from build123d import *

# Parameters (mm, degrees)
CYLINDER009_R     = 1.75
CYLINDER009_DEPTH = 10
CYLINDER010_R     = 2.5
CYLINDER010_DEPTH = 4
CYLINDER008_R     = 1.75
CYLINDER008_DEPTH = 10
CYLINDER011_R     = 2.5
CYLINDER011_DEPTH = 4
CYLINDER007_R     = 1.75
CYLINDER007_DEPTH = 10
CYLINDER013_R     = 2.5
CYLINDER013_DEPTH = 4
CYLINDER006_R     = 1.75
CYLINDER006_DEPTH = 10
CYLINDER012_R     = 2.5
CYLINDER012_DEPTH = 4
CYLINDER005_R     = 1.75
CYLINDER005_DEPTH = 10
CYLINDER014_R     = 2.5
CYLINDER014_DEPTH = 4
CYLINDER004_R     = 1.75
CYLINDER004_DEPTH = 10
CYLINDER015_R     = 2.5
CYLINDER015_DEPTH = 4
CYLINDER003_R     = 1
CYLINDER003_DEPTH = 10
CYLINDER002_R     = 1
CYLINDER002_DEPTH = 10
CYLINDER001_R     = 1
CYLINDER001_DEPTH = 10
CYLINDER_R        = 1
CYLINDER_DEPTH    = 10
BOX001_W          = 72
BOX001_H          = 25
BOX001_DEPTH      = 10
BOX_W             = 86
BOX_H             = 70
BOX_DEPTH         = 2
CHAMFER_SIZE      = 0.5
CHAMFER001_SIZE   = 0.5


with BuildPart() as cilindro009:
    # Cylinder009 → Cylinder009 (new body)
    with BuildSketch(Plane(origin=(42, 12.5, -3), x_dir=(1, 0, 0), z_dir=(0, 0, 1))):
        Circle(CYLINDER009_R)
    extrude(amount=CYLINDER009_DEPTH)


with BuildPart() as cut011:
    # Cylinder010 → Cylinder010 (new body)
    with BuildSketch(Plane(origin=(42, 12.5, -2), x_dir=(1, 0, 0), z_dir=(0, 0, 1))):
        Circle(CYLINDER010_R)
    extrude(amount=CYLINDER010_DEPTH)

    # Cut011: cut Cilindro009
    add(cilindro009.part, mode=Mode.SUBTRACT)


with BuildPart() as cilindro008:
    # Cylinder008 → Cylinder008 (new body)
    with BuildSketch(Plane(origin=(34.5, 12.5, -3), x_dir=(1, 0, 0), z_dir=(0, 0, 1))):
        Circle(CYLINDER008_R)
    extrude(amount=CYLINDER008_DEPTH)


with BuildPart() as cut012:
    # Cylinder011 → Cylinder011 (new body)
    with BuildSketch(Plane(origin=(34.5, 12.5, -2), x_dir=(1, 0, 0), z_dir=(0, 0, 1))):
        Circle(CYLINDER011_R)
    extrude(amount=CYLINDER011_DEPTH)

    # Cut012: cut Cilindro008
    add(cilindro008.part, mode=Mode.SUBTRACT)


with BuildPart() as cilindro007:
    # Cylinder007 → Cylinder007 (new body)
    with BuildSketch(Plane(origin=(25, 9.5, -3), x_dir=(1, 0, 0), z_dir=(0, 0, 1))):
        Circle(CYLINDER007_R)
    extrude(amount=CYLINDER007_DEPTH)


with BuildPart() as cut013:
    # Cylinder013 → Cylinder013 (new body)
    with BuildSketch(Plane(origin=(25, 9.5, -2), x_dir=(1, 0, 0), z_dir=(0, 0, 1))):
        Circle(CYLINDER013_R)
    extrude(amount=CYLINDER013_DEPTH)

    # Cut013: cut Cilindro007
    add(cilindro007.part, mode=Mode.SUBTRACT)


with BuildPart() as cilindro006:
    # Cylinder006 → Cylinder006 (new body)
    with BuildSketch(Plane(origin=(25, 16.5, -3), x_dir=(1, 0, 0), z_dir=(0, 0, 1))):
        Circle(CYLINDER006_R)
    extrude(amount=CYLINDER006_DEPTH)


with BuildPart() as cut014:
    # Cylinder012 → Cylinder012 (new body)
    with BuildSketch(Plane(origin=(25, 16.5, -2), x_dir=(1, 0, 0), z_dir=(0, 0, 1))):
        Circle(CYLINDER012_R)
    extrude(amount=CYLINDER012_DEPTH)

    # Cut014: cut Cilindro006
    add(cilindro006.part, mode=Mode.SUBTRACT)


with BuildPart() as cilindro005:
    # Cylinder005 → Cylinder005 (new body)
    with BuildSketch(Plane(origin=(15, 12.5, -3), x_dir=(1, 0, 0), z_dir=(0, 0, 1))):
        Circle(CYLINDER005_R)
    extrude(amount=CYLINDER005_DEPTH)


with BuildPart() as cut015:
    # Cylinder014 → Cylinder014 (new body)
    with BuildSketch(Plane(origin=(15, 12.5, -2), x_dir=(1, 0, 0), z_dir=(0, 0, 1))):
        Circle(CYLINDER014_R)
    extrude(amount=CYLINDER014_DEPTH)

    # Cut015: cut Cilindro005
    add(cilindro005.part, mode=Mode.SUBTRACT)


with BuildPart() as cilindro004:
    # Cylinder004 → Cylinder004 (new body)
    with BuildSketch(Plane(origin=(7.5, 12.5, -3), x_dir=(1, 0, 0), z_dir=(0, 0, 1))):
        Circle(CYLINDER004_R)
    extrude(amount=CYLINDER004_DEPTH)


with BuildPart() as cut016:
    # Cylinder015 → Cylinder015 (new body)
    with BuildSketch(Plane(origin=(7.5, 12.5, -2), x_dir=(1, 0, 0), z_dir=(0, 0, 1))):
        Circle(CYLINDER015_R)
    extrude(amount=CYLINDER015_DEPTH)

    # Cut016: cut Cilindro004
    add(cilindro004.part, mode=Mode.SUBTRACT)


with BuildPart() as cilindro003:
    # Cylinder003 → Cylinder003 (new body)
    with BuildSketch(Plane(origin=(83, 67, -1), x_dir=(1, 0, 0), z_dir=(0, 0, 1))):
        Circle(CYLINDER003_R)
    extrude(amount=CYLINDER003_DEPTH)


with BuildPart() as cilindro002:
    # Cylinder002 → Cylinder002 (new body)
    with BuildSketch(Plane(origin=(83, 3, -1), x_dir=(1, 0, 0), z_dir=(0, 0, 1))):
        Circle(CYLINDER002_R)
    extrude(amount=CYLINDER002_DEPTH)


with BuildPart() as cilindro001:
    # Cylinder001 → Cylinder001 (new body)
    with BuildSketch(Plane(origin=(3, 67, -1), x_dir=(1, 0, 0), z_dir=(0, 0, 1))):
        Circle(CYLINDER001_R)
    extrude(amount=CYLINDER001_DEPTH)


with BuildPart() as cilindro:
    # Cylinder → Cylinder (new body)
    with BuildSketch(Plane(origin=(3, 3, -1), x_dir=(1, 0, 0), z_dir=(0, 0, 1))):
        Circle(CYLINDER_R)
    extrude(amount=CYLINDER_DEPTH)


with BuildPart() as cubo001:
    # Box001 → Box001 (new body)
    with BuildSketch(Plane(origin=(7, 25.5, 0), x_dir=(1, 0, 0), z_dir=(0, 0, 1))):
        with Locations((36, 12.5)):
            Rectangle(BOX001_W, BOX001_H)
    extrude(amount=BOX001_DEPTH)


with BuildPart() as fusion001:
    # Box → Box (new body)
    with BuildSketch(Plane.XY):
        with Locations((43, 35)):
            Rectangle(BOX_W, BOX_H)
    extrude(amount=BOX_DEPTH)

    # Cut: cut Cubo001
    add(cubo001.part, mode=Mode.SUBTRACT)

    # Cut001: cut Cilindro
    add(cilindro.part, mode=Mode.SUBTRACT)

    # Cut002: cut Cilindro001
    add(cilindro001.part, mode=Mode.SUBTRACT)

    # Cut003: cut Cilindro002
    add(cilindro002.part, mode=Mode.SUBTRACT)

    # Cut004: cut Cilindro003
    add(cilindro003.part, mode=Mode.SUBTRACT)

    # Cut005: cut Cilindro004
    add(cilindro004.part, mode=Mode.SUBTRACT)

    # Cut006: cut Cilindro005
    add(cilindro005.part, mode=Mode.SUBTRACT)

    # Cut007: cut Cilindro006
    add(cilindro006.part, mode=Mode.SUBTRACT)

    # Cut008: cut Cilindro007
    add(cilindro007.part, mode=Mode.SUBTRACT)

    # Cut009: cut Cilindro008
    add(cilindro008.part, mode=Mode.SUBTRACT)

    # Cut010: cut Cilindro009
    add(cilindro009.part, mode=Mode.SUBTRACT)

    # Chamfer
    chamfer_edges = [fusion001.edges().sort_by_distance(p)[0] for p in [
        (0, 35, 2),
        (43, 0, 2),
        (43, 70, 2),
        (86, 35, 2),
        (43, 25.5, 2),
        (79, 38, 2),
        (7, 38, 2),
        (43, 50.5, 2),
    ]]
    chamfer(chamfer_edges, length=CHAMFER_SIZE)

    # Chamfer001
    chamfer001_edges = [fusion001.edges().sort_by_distance(p)[0] for p in [
        (2, 3, 2),
        (82, 3, 2),
        (2, 67, 2),
        (82, 67, 2),
    ]]
    chamfer(chamfer001_edges, length=CHAMFER001_SIZE)

    # Fusion: union Cut011, Cut012, Cut013, Cut014, Cut015, Cut016
    add(cut011.part)
    add(cut012.part)
    add(cut013.part)
    add(cut014.part)
    add(cut015.part)
    add(cut016.part)


solid = fusion001.part
Read the model definition and answer for the solid it produces. Units are mm, in the model's axes. A direction names the side the tool comes from. Coordinates: 2 decimals unless noted, no trailing zeros. Order: outer loops, then holes, each group sorted by start corner. A loop starts at its lowest first (then second) coordinate and runs counter-clockwise, first axis right, second up. Notation, with made-up numbers: (83, 61.5) -> (108, 61.5) arc R16 cw to (108, 88.5) -> close; hole circle Ø4 at (22.25, -3.75). An arc over 180 degrees is marked (long way). Answer as a JSON object with one key per item and string values.
1) A cutting plane is placed at B-B, the plane y = 36. Determine the outline of the cut face in (x, z), plus the area to 3 significant figures.
Model answer:
{"outline": "(0, 0) -> (7, 0) -> (7, 1.5) -> (6.5, 2) -> (0.5, 2) -> (0, 1.5) -> close; (79, 0) -> (86, 0) -> (86, 1.5) -> (85.5, 2) -> (79.5, 2) -> (79, 1.5) -> close", "area": "27.5 mm²"}
2) A cutting plane is placed at C-C, the plane y = 67. Determine the outline of the cut face in (x, z), plus the area to 3 significant figures.
Model answer:
{"outline": "(0, 0) -> (2, 0) -> (2, 1.5) -> (1.5, 2) -> (0.5, 2) -> (0, 1.5) -> close; (4, 0) -> (82, 0) -> (82, 1.5) -> (81.5, 2) -> (4.5, 2) -> (4, 1.5) -> close; (84, 0) -> (86, 0) -> (86, 1.5) -> (85.5, 2) -> (84.5, 2) -> (84, 1.5) -> close", "area": "163 mm²"}
3) A cutting plane is placed at D-D, the plane y = 53. Determine the outline of the cut face in (x, z).
Model answer:
{"outline": "(0, 0) -> (86, 0) -> (86, 1.5) -> (85.5, 2) -> (0.5, 2) -> (0, 1.5) -> close"}
4) The mould has two halves that part along Y. Classify faces 1 (the face through (8.65, 10.28, -1.01)), 2 (the face through (23, 16, -2)), 3 (the face through (3, 66, 1)), 4 (the face through (43.617, 11.83, -0.028)): released by +Y, released by -Y, zero draft, split by the parting line, or undercut.
Model answer:
{"face 1": "split by the parting line", "face 2": "zero draft", "face 3": "undercut", "face 4": "undercut"}
5) A cutting plane is placed at A-A, the plane x = 11. Determine the outline of the cut face in (y, z), plus the area to 3 significant figures.
Model answer:
{"outline": "(0, 0) -> (25.5, 0) -> (25.5, 1.5) -> (25, 2) -> (0.5, 2) -> (0, 1.5) -> close; (50.5, 0) -> (70, 0) -> (70, 1.5) -> (69.5, 2) -> (51, 2) -> (50.5, 1.5) -> close", "area": "89.5 mm²"}
6) Each of these flat-tipped pins is pushed along its axis until it touches: pin 1 (2 mm diameter, centred on x = 42, y = 12.5, fed in from +Z); pin 2 (2.5 mm diameter, centred on x = 83, y = 67, fed in from +Z). Where does it stop, or does it pass through?
Model answer:
{"pin 1": "passes through", "pin 2": "stops at z = 1.75"}
7) A tool of negligible diameter and unlimited length cuts with its end or side. For faces 5 (the face through (9, 11, -2)), 6 (the face through (22.5, 16.6, -1)), from which of +Z, -Z, +X, -X, +Y, -Y can it reach the whole face along a straight path? Write none if from no direction.
Model answer:
{"face 5": "-Z, +X, -X, +Y, -Y", "face 6": "-Z"}
8) Consider line 1 along Y through (x, z) = (3, 0.8); line 2 along Y through (x, z) = (25, 1); line 3 along X through (y, z) = (3, 0.8). Determine where each line is inside the solid, lowest interval first. Write a range as from..to.
Model answer:
{"line 1": "y = 0..2, 4..66, 68..70", "line 2": "y = 0..7.75, 11.25..14.75, 18.25..25.5, 50.5..70", "line 3": "x = 0..2, 4..82, 84..86"}
